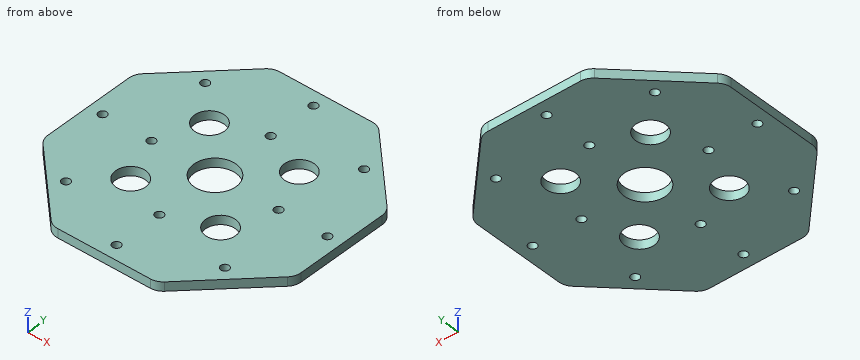
from build123d import *

# Parameters (mm, degrees)
F0_R     = 1.4
F0_R_2   = 5
F0_R_3   = 7
F1_DEPTH = 3


with BuildPart() as f1:
    # F0 (on Top) → F1 (new body)
    with BuildSketch(Plane.XY):
        with BuildLine():
            Line((15.428932, 42.248737), (-15.428932, 42.248737))
            ThreePointArc((-15.428932, 42.248737), (-17.342349, 41.868135), (-18.964466, 40.784271))
            Line((-18.964466, 40.784271), (-40.784271, 18.964466))
            ThreePointArc((-40.784271, 18.964466), (-41.868135, 17.342349), (-42.248737, 15.428932))
            Line((-42.248737, 15.428932), (-42.248737, -15.428932))
            ThreePointArc((-42.248737, -15.428932), (-41.868135, -17.342349), (-40.784271, -18.964466))
            Line((-40.784271, -18.964466), (-18.964466, -40.784271))
            ThreePointArc((-18.964466, -40.784271), (-17.342349, -41.868135), (-15.428932, -42.248737))
            Line((-15.428932, -42.248737), (15.428932, -42.248737))
            ThreePointArc((15.428932, -42.248737), (17.342349, -41.868135), (18.964466, -40.784271))
            Line((18.964466, -40.784271), (40.784271, -18.964466))
            ThreePointArc((40.784271, -18.964466), (41.868135, -17.342349), (42.248737, -15.428932))
            Line((42.248737, -15.428932), (42.248737, 15.428932))
            ThreePointArc((42.248737, 15.428932), (41.868135, 17.342349), (40.784271, 18.964466))
            Line((40.784271, 18.964466), (18.964466, 40.784271))
            ThreePointArc((18.964466, 40.784271), (17.342349, 41.868135), (15.428932, 42.248737))
        make_face()
        with Locations((-26.516504, -26.516504)):
            Circle(F0_R, mode=Mode.SUBTRACT)
        with Locations((0, -37.5)):
            Circle(F0_R, mode=Mode.SUBTRACT)
        with Locations((0, -21.213203)):
            Circle(F0_R, mode=Mode.SUBTRACT)
        with Locations((-37.5, 0)):
            Circle(F0_R, mode=Mode.SUBTRACT)
        with Locations((-21.213203, 0)):
            Circle(F0_R, mode=Mode.SUBTRACT)
        with Locations((-15, -15)):
            Circle(F0_R_2, mode=Mode.SUBTRACT)
        Circle(F0_R_3, mode=Mode.SUBTRACT)
        with Locations((26.516504, -26.516504)):
            Circle(F0_R, mode=Mode.SUBTRACT)
        with Locations((15, -15)):
            Circle(F0_R_2, mode=Mode.SUBTRACT)
        with Locations((21.213203, 0)):
            Circle(F0_R, mode=Mode.SUBTRACT)
        with Locations((37.5, 0)):
            Circle(F0_R, mode=Mode.SUBTRACT)
        with Locations((-15, 15)):
            Circle(F0_R_2, mode=Mode.SUBTRACT)
        with Locations((-26.516504, 26.516504)):
            Circle(F0_R, mode=Mode.SUBTRACT)
        with Locations((0, 21.213203)):
            Circle(F0_R, mode=Mode.SUBTRACT)
        with Locations((0, 37.5)):
            Circle(F0_R, mode=Mode.SUBTRACT)
        with Locations((15, 15)):
            Circle(F0_R_2, mode=Mode.SUBTRACT)
        with Locations((26.516504, 26.516504)):
            Circle(F0_R, mode=Mode.SUBTRACT)
    extrude(amount=F1_DEPTH)


solid = f1.part
Source: CAD feature listing. Evaluate the final solid. Frame: model axes, mm. Round coordinates to 2 decimals unless told otherwise and drop trailing zeros. Loops run counter-clockwise (first coordinate to the right, second up) from the corner with the lowest first, then second, coordinate; pieces in that order, holes last.
Q1. Section D-D, the plane y = -37.5. Return loops of the section in (x, z), plus the area to 3 significant figures.
Q2. Section B-B, the plane x = 5.5. Return loops of the section in (y, z), plus the area to 3 significant figures.
Q3. Section A-A, the plane y = 0. Return loops of the section in (x, z), plus the area to 3 significant figures.
Q4. First-contact query: P1, Ø1, axis at x = -23, z = 1.5, coming from the -Y side; P2, Ø1.5, axis at x = 27.5, z = 1, coming from the +Y side. Flat tips, straight axial feed; report the tip coordinate or a pass-through.
Q5. Ray query, line 1 (Y direction, x = 0, z = 0.8); line 2 (X direction, y = 12, z = 1.9); line 3 (X direction, y = -17.5, z = 0.55). Return the intervals inside material, ascending.
Q6. Section C-C, the plane z = 2. State how many separate pieces and enclosed holes the cut face has, plus the area to 3 significant figures.
Solutions:
1. outline: (-22.25, 0) - (-1.4, 0) - (-1.4, 3) - (-22.25, 3) - close; (1.4, 0) - (22.25, 0) - (22.25, 3) - (1.4, 3) - close
1. area: 125 mm2
2. outline: (-42.25, 0) - (-4.33, 0) - (-4.33, 3) - (-42.25, 3) - close; (4.33, 0) - (42.25, 0) - (42.25, 3) - (4.33, 3) - close
2. area: 228 mm2
3. outline: (-42.25, 0) - (-38.9, 0) - (-38.9, 3) - (-42.25, 3) - close; (-36.1, 0) - (-22.61, 0) - (-22.61, 3) - (-36.1, 3) - close; (-19.81, 0) - (-7, 0) - (-7, 3) - (-19.81, 3) - close; (7, 0) - (19.81, 0) - (19.81, 3) - (7, 3) - close; (22.61, 0) - (36.1, 0) - (36.1, 3) - (22.61, 3) - close; (38.9, 0) - (42.25, 0) - (42.25, 3) - (38.9, 3) - close
3. area: 178 mm2
4. P1: stops at y = -37.25
4. P2: stops at y = 33
5. line 1: y = -42.25 to -38.9, -36.1 to -22.61, -19.81 to -7, 7 to 19.81, 22.61 to 36.1, 38.9 to 42.25
5. line 2: x = -42.25 to -19, -11 to 11, 19 to 42.25
5. line 3: x = -41.8 to -19.33, -10.67 to 10.67, 19.33 to 41.8
6. separate pieces: 1
6. enclosed holes: 17
6. area: 5,370 mm2
